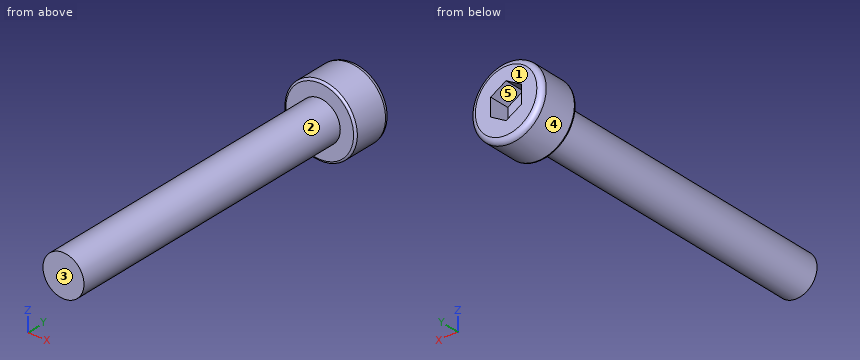
Autodesk Inventor part; units mm, degrees
ref_plane "YZ Plane" through (0, 0, 0) normal (1, 0, 0) x (0, 1, 0)
ref_plane "XZ Plane" through (0, 0, 0) normal (0, 1, 0) x (-1, 0, 0)
ref_plane "XY Plane" through (0, 0, 0) normal (0, 0, 1) x (1, 0, 0)
sketch "スケッチ1" plane through (0, 0, 0) normal (0, 1, 0) x (-1, 0, 0)
  circle A0 centre (0, 0) radius 3.5
  dimension "d0" = 7
extrude "押し出し1" add sketch "スケッチ1" along normal blind 4
sketch "スケッチ2" plane through (0, 0, 0) normal (0, -1, 0) x (1, 0, 0)
  circle A0 centre (0, 0) radius 2
  dimension "d3" = 4
extrude "押し出し2" add sketch "スケッチ2" along normal blind 30
fillet "フィレット1" radius 0.5 1 edges at (3.5, 4, 0)
fillet "フィレット1" radius 0.2 1 edges at (3.5, 0, 0)
sketch "スケッチ3" plane through (0, 4, 0) normal (0, 1, 0) x (1, 0, 0)
  line L0 (0, 1.7321) -> (-1.5, 0.866)
  line L1 (-1.5, 0.866) -> (-1.5, -0.866)
  line L2 (-1.5, -0.866) -> (0, -1.7321)
  line L3 (0, -1.7321) -> (1.5, -0.866)
  line L4 (1.5, -0.866) -> (1.5, 0.866)
  line L5 (1.5, 0.866) -> (0, 1.7321)
  line L6 (0, 1.7321) -> (0, -1.7321) construction
  circle A0 centre (0, 0) radius 1.7321 construction
  dimension "d12" = 3
extrude "押し出し3" cut sketch "スケッチ3" against normal blind 2
thread "ねじ1"
properties part number "M3-CapScrew"
Here's how the part is built. I have some questions about the finished solid (model axes, mm). Face numbers are marked on the shaded views. A direction names the side the tool comes from. Coordinates: 2 decimals unless noted, no trailing zeros. Order: outer loops, then holes, each group sorted by start corner. A loop starts at its lowest first (then second) coordinate and runs counter-clockwise, first axis right, second up.
1) We'd pull the mould along X, two halves only. Please class the marked faces 3, 4 and 5: +X half, -X half, draft (parallel to the pull), parting line (faces both ways), or undercut.
2) Will these pins go through, and if not, where does the flat tip stop? pin 1 (4 mm diameter, centred on x = -2.5, y = -13, fed in from -Z); pin 2 (1 mm diameter, centred on y = -16, z = -0.5, fed in from -X); pin 3 (0.9 mm diameter, centred on x = -0.5, z = 0, fed in from +Y).
3) Imagine slicing it at A-A on z = 0. List the corners of the cut face in (x, y) for me, and give its area (3 significant figures).
4) I need wall thicknesses on line 1 (Z direction, x = 0.5, y = 2.5); line 2 (Y direction, x = 1.75, z = 1.5); line 3 (Y direction, x = -0.25, z = -1). Which ranges of each line are inside material? Lowest first, please.
5) Which directions (+Z, -Z, +X, -X, +Y, -Y) give clear straight access to the entire face, cutting with the end or side of a thin tool? Please do the marked faces 1 and 2.
6) Imagine slicing it at B-B on y = -10. List the corners of the cut face in (x, z) for me.
Response values:
1. face 3: draft
1. face 4: parting line
1. face 5: undercut
2. pin 1: stops at z = -1.94
2. pin 2: stops at x = -2
2. pin 3: stops at y = 2
3. outline: (-3.5, 0.2) arc R0.2 ccw to (-3.3, 0) - (-2, 0) - (-2, -30) - (2, -30) - (2, 0) - (3.3, 0) arc R0.2 ccw to (3.5, 0.2) - (3.5, 3.5) arc R0.5 ccw to (3, 4) - (1.5, 4) - (1.5, 2) - (-1.5, 2) - (-1.5, 4) - (-3, 4) arc R0.5 ccw to (-3.5, 3.5) - close
3. area: 142 mm2
4. line 1: z = -3.46 to -1.44, 1.44 to 3.46
4. line 2: y = 0 to 4
4. line 3: y = -30 to 2
5. face 1: +Z, -Z, +X, -X, +Y
5. face 2: -Y
6. outline: circle Ø4 at (0, 0)
